```python
from build123d import *

# Parameters (mm, degrees)
SKETCH1_R           = 1.5
BOSS_EXTRUDE1_DEPTH = 3


with BuildPart() as part:
    # Sketch1 → Boss-Extrude1 (new body)
    with BuildSketch(Plane(origin=(0, 0, 0), x_dir=(0, 0, -1), z_dir=(1, 0, 0))):
        Polygon((15, 3.289322104), (-15, 3.289322104), (-15, 22.289322104), (-18, 22.289322104), (-18, 32.289322104), (-15, 32.289322104), (15, 32.289322104), (18, 32.289322104), (18, 22.289322104), (15, 22.289322104), align=None)
        with Locations((7.94, 11.619322104)):
            Circle(SKETCH1_R, mode=Mode.SUBTRACT)
        with Locations(Location((-7.94, 11.619322104, 0), (0, 0, 180))):
            Circle(SKETCH1_R, mode=Mode.SUBTRACT)
        with Locations((11, 26.789322104)):
            Circle(SKETCH1_R, mode=Mode.SUBTRACT)
        with Locations(Location((-11, 26.789322104, 0), (0, 0, 180))):
            Circle(SKETCH1_R, mode=Mode.SUBTRACT)
    extrude(amount=BOSS_EXTRUDE1_DEPTH)


solid = part.part
```
Part model, mm, in its own coordinate system. A direction names the side the tool comes from. Give positions to 0.01 mm unless a question says otherwise; leave off trailing zeros. Write each loop counter-clockwise with the first axis right and the second up, starting at its lowest first coordinate (ties: lowest second). Pieces come first, ordered by that corner, then holes. Notation, with made-up numbers: M 11.5,50 L 39.5,50 A25 cw 39.5,88 Z; hole C 23.5,-16.75 d4. An arc over 180 degrees is marked long. Use CSV: the item, a comma, the result in double quotes.
Item 1: Which spindle directions (+Z, -Z, +X, -X, +Y, -Y) get a long thin tool onto all of the face, cutting with end or side? Do faces 1 (the face through (1, 22.289, 16)), 2 (the face through (1.479, 25.325, -10.675)), 3 (the face through (1, 22.289, -17)). Say none if no direction does.
Taken from the geometry:
face 1,"+Z, +X, -X, -Y"
face 2,"+X, -X"
face 3,"-Z, +X, -X, -Y"
Item 2: Slice it at D-D on y = 18.25. Write the cut outline in (x, z), plus the area to 3 significant figures.
Taken from the geometry:
outline,"M 0,-15 L 3,-15 L 3,15 L 0,15 Z"
area,"90.0 mm²"
Item 3: Pin check, flat tips, straight feed: P1, Ø5, axis at y = 11.62, z = -7.94, coming from the +X side; P2, Ø0.9, axis at x = 2, z = -17, coming from the -Y side. Stop position of each tip, or through.
Taken from the geometry:
P1,"stops at x = 3"
P2,"stops at y = 22.29"
Item 4: Slice it at C-C on x = 0.95. Write the cut outline in (y, z).
Taken from the geometry:
outline,"M 3.29,-15 L 22.29,-15 L 22.29,-18 L 32.29,-18 L 32.29,18 L 22.29,18 L 22.29,15 L 3.29,15 Z; hole C 11.62,-7.94 d3; hole C 11.62,7.94 d3; hole C 26.79,-11 d3; hole C 26.79,11 d3"
Item 5: Slice it at B-B on y = 12.25. Write the cut outline in (x, z), plus the area to 3 significant figures.
Taken from the geometry:
outline,"M 0,-15 L 3,-15 L 3,-9.3 L 0,-9.3 Z; M 0,-6.58 L 3,-6.58 L 3,6.58 L 0,6.58 Z; M 0,9.3 L 3,9.3 L 3,15 L 0,15 Z"
area,"73.7 mm²"
Item 6: Drill centre lines: probe 1 along Z at (x, y) = (1.4, 26.75); probe 2 along Z at (x, y) = (2.25, 11.5); probe 3 along Y at (x, z) = (2.1, -11). Where is each one in solid material? Low to high.
Taken from the geometry:
probe 1,"z = -18 to -12.5, -9.5 to 9.5, 12.5 to 18"
probe 2,"z = -15 to -9.44, -6.44 to 6.44, 9.44 to 15"
probe 3,"y = 3.29 to 25.29, 28.29 to 32.29"
Item 7: Pull direction Y, two halves, no side cores. Call faces 4 (the face through (1, 3.289, 0)), 5 (the face through (1.479, 13.084, 7.615)), 6 (the face through (3, 18, 0)): +Y half, -Y half, draft (parallel to the pull), parting line (faces both ways), or undercut.
Taken from the geometry:
face 4,"-Y half"
face 5,"undercut"
face 6,"draft"
Item 8: Slice it at A-A on z = -7.94. Write the cut outline in (x, y).
Taken from the geometry:
outline,"M 0,3.29 L 3,3.29 L 3,10.12 L 0,10.12 Z; M 0,13.12 L 3,13.12 L 3,32.29 L 0,32.29 Z"
